Input: dimensioned drawing with shaded views. Units: mm. Origin: part minimum x, y, z. A direction names the side the tool comes from. Give positions to 0.01 mm unless a question says otherwise; leave off trailing zeros. Loops run counter-clockwise (first coordinate to the right, second up) from the corner with the lowest first, then second, coordinate; pieces in that order, holes last.
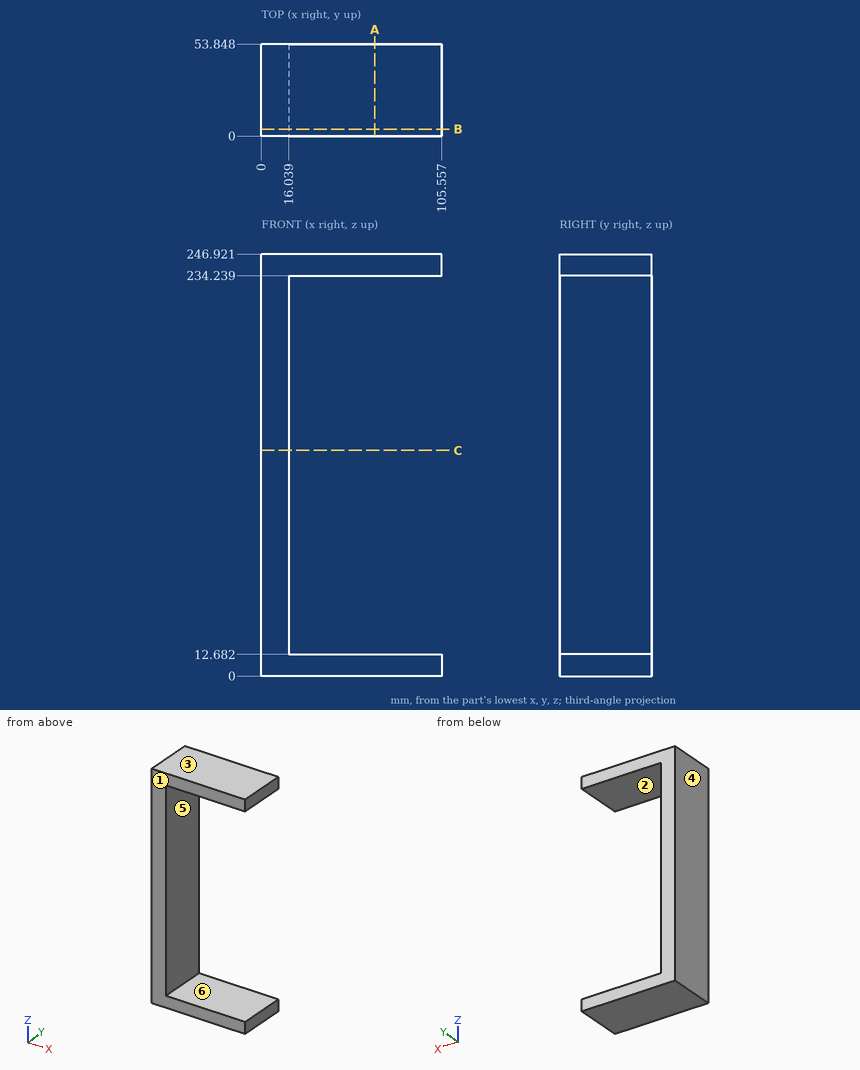
Item 1: Draft query along Z for the marked faces 3, 4, 5 and 6. Return one class per face: +Z half, -Z half, draft (parallel to the pull), parting line (faces both ways), or undercut.
Values follow:
face 3: +Z half
face 4: draft
face 5: undercut
face 6: undercut
Item 2: Section query B-B on y = 4. Return loops of the section in (x, z), plus the area to 3 significant figures.
Values follow:
outline: (0, 0) - (105.56, 0) - (105.56, 12.68) - (16.04, 12.68) - (16.04, 234.24) - (105.56, 234.24) - (105.56, 246.92) - (0, 246.92) - close
area: 6,230 mm2
Item 3: Section query C-C on z = 132. Return loops of the section in (x, y), plus the area to 3 significant figures.
Values follow:
outline: (0, 0) - (16.04, 0) - (16.04, 53.85) - (0, 53.85) - close
area: 864 mm2
Item 4: Ray query, probe 1 along Z at (x, y) = (45, 25.5); probe 2 along X at (y, z) = (36, 222.5). Return the intervals inside material, ascending.
Values follow:
probe 1: z = 0 to 12.68, 234.24 to 246.92
probe 2: x = 0 to 16.04
Item 5: Set-up query: the marked faces 1 and 2. Return all of +Z, -Z, +X, -X, +Y, -Y with unobstructed straight access to the full face (end or side cutting, diameter ignored); none if empty.
Values follow:
face 1: +Z, -Z, +X, -X, -Y
face 2: +X, +Y, -Y
Item 6: Section query A-A on x = 66.5. Return loops of the section in (y, z), plus the area to 3 significant figures.
Values follow:
outline: (0, 0) - (53.85, 0) - (53.85, 12.68) - (0, 12.68) - close; (0, 234.24) - (53.85, 234.24) - (53.85, 246.92) - (0, 246.92) - close
area: 1,370 mm2
Item 7: Pin query (flat end, axial travel): pin 1 (16 mm diameter, centred on y = 18.5, z = 142, fed in from +X). Return the tip coordinate at first contact, or that it passes through.
Values follow:
pin 1: stops at x = 16.04
